The drawing under review shows one solid part. Ordinate dimensions are in mm from its lowest x, y, z. Coordinates: 2 decimals unless noted, no trailing zeros. Write each loop counter-clockwise with the first axis right and the second up, starting at its lowest first coordinate (ties: lowest second). Pieces come first, ordered by that corner, then holes. Notation, with made-up numbers: M 31,12.25 L 40,12.25 A22 ccw 40,21.25 Z; hole C 88,-18.5 d11. An arc over 180 degrees is marked long. Write each question's results on one line, items separated by ' | '. Start each with the question number.
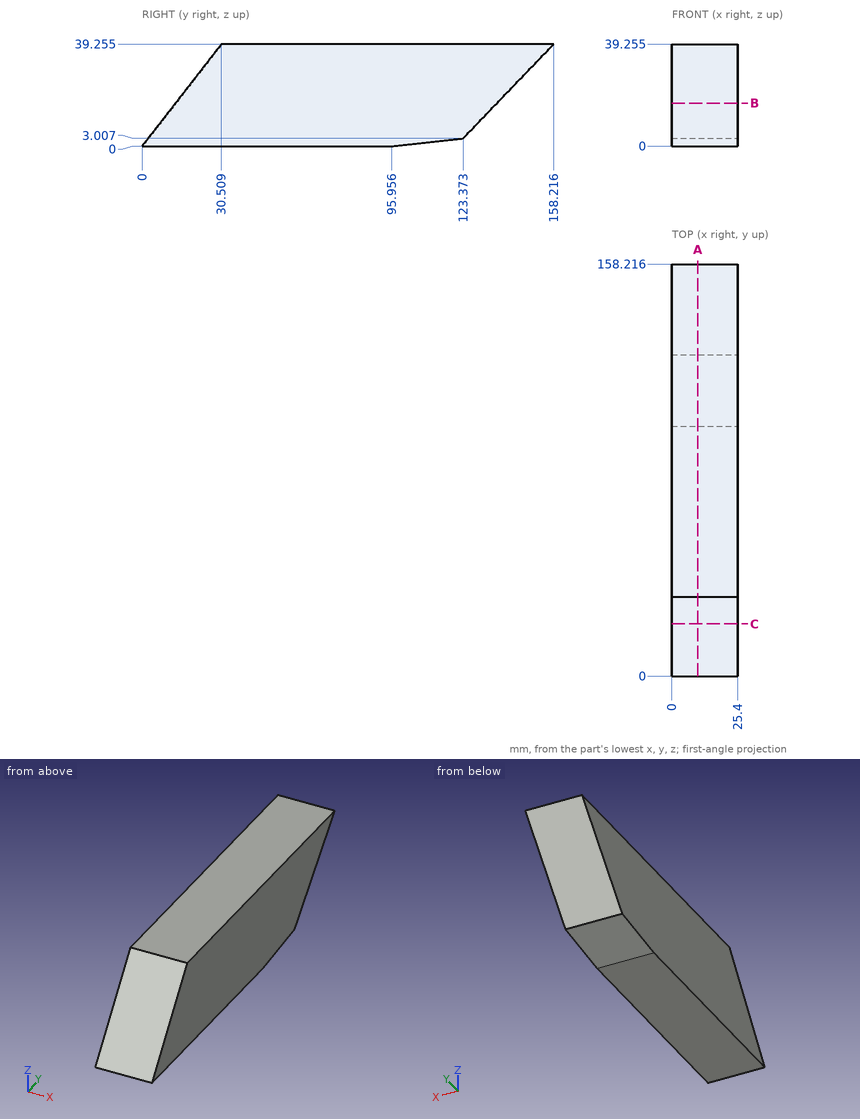
Item 1: We need section A-A on x = 10. State the section outline as (y, z) points (1 decimal).
Item 2: Insertion check: pin 1 Ø1.5 at (x, z) = (9, 8.5) entering from -Y; pin 2 Ø6 at (x, z) = (3, 28.5) entering from +Y; pin 3 Ø12 at (x, y) = (18, 128) entering from -Z. Each pin has a flat end and moves straight along its axis. Give the tip position at first contact, or say it passes through.
Item 3: We need section C-C on y = 20. State the section outline as (x, z) points.
Item 4: We need section B-B on z = 16.5. State the section outline as (x, y) points.
Item 5: Wall thickness on L1, parallel to Z at x = 21.75, y = 138 (1 decimal); L2, parallel to Y at x = 7.75, z = 18 (1 decimal); L3, parallel to Y at x = 3.25, z = 21: over which ranges is each line inside the solid? List them lowest first.
Answer:
1) outline: M 0,0 L 96,0 L 123.4,3 L 158.2,39.3 L 30.5,39.3 Z
2) pin 1: stops at y = 6.02 | pin 2: stops at y = 150.76 | pin 3: stops at z = 2.86
3) outline: M 0,0 L 25.4,0 L 25.4,25.73 L 0,25.73 Z
4) outline: M 0,12.82 L 25.4,12.82 L 25.4,136.34 L 0,136.34 Z
5) L1: z = 18.2 to 39.3 | L2: y = 14 to 137.8 | L3: y = 16.32 to 140.67
